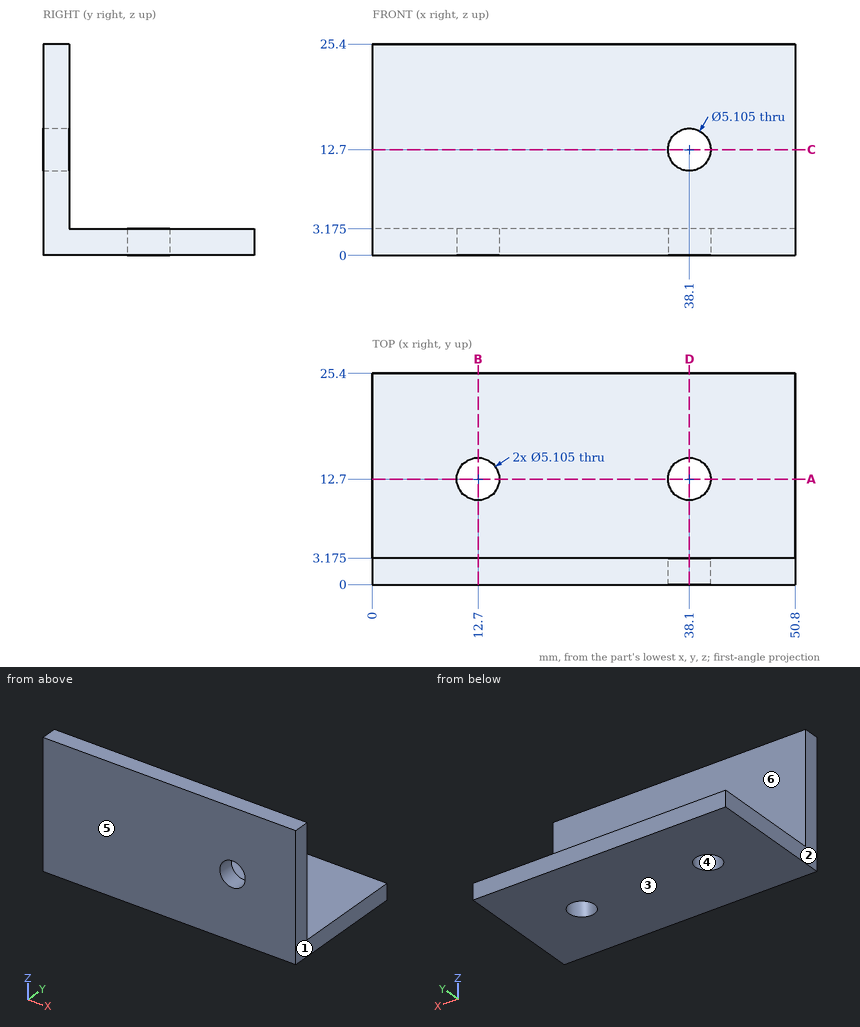
Input: dimensioned drawing with shaded views. Units: mm. Origin: part minimum x, y, z. A direction names the side the tool comes from. Give positions to 0.01 mm unless a question says otherwise; leave off trailing zeros. Loops run counter-clockwise (first coordinate to the right, second up) from the corner with the lowest first, then second, coordinate; pieces in that order, holes last. Notation, with made-up numbers: M 37.5,13.25 L 71.5,13.25 A19 cw 71.5,40.25 Z; hole C 25,68.25 d6. An arc over 180 degrees is marked long. Put each result on its own line as item: value. Start each with the question number.
1) Pull-direction query (X, two-part tool) for the marked faces 1, 2, 3 and 4; classes: pulls with the +X half, pulls with the -X half, needs draft (parallel to the pull), parting line crosses it, or undercut.
2) Cut plane A-A (y = 12.7). Output: boundary loops of the cut face in (x, z) (1 decimal), then the cut area to 3 significant figures.
3) Cut plane C-C (z = 12.7). Output: boundary loops of the cut face in (x, y) (1 decimal).
4) Cut plane D-D (x = 38.1). Output: boundary loops of the cut face in (y, z) (1 decimal), then the cut area to 3 significant figures.
5) Contact query for flat-ended pins moving along their axis: pin 1 (2 mm diameter, centred on x = 38, y = 6, fed in from +Z) (3 decimals); pin 2 (8 mm diameter, centred on y = 5.5, z = 18, fed in from -X); pin 3 (1 mm diameter, centred on y = 16, z = 4.5, fed in from +X); pin 4 (1 mm diameter, centred on x = 43, z = 14, fed in from +Y) (3 decimals). Output: stop coordinate, or through.
6) Cut plane B-B (x = 12.7). Output: boundary loops of the cut face in (y, z) (1 decimal).
7) Ray query, line 1 along Y through (x, z) = (38.1, 2); line 2 along Z through (x, y) = (41, 23.75) (1 decimal). Return the intervals inside material, ascending.
8) Access query for the marked faces 5 and 6. Directions: +Z, -Z, +X, -X, +Y, -Y. A direction counts if a zero-diameter tool reaches every point of the face in a straight line with its end or side. Return the directions, or none.
Verdict:
1. face 1: pulls with the +X half
1. face 2: pulls with the -X half
1. face 3: needs draft
1. face 4: undercut
2. outline: M 0,0 L 10.1,0 L 10.1,3.2 L 0,3.2 Z; M 15.3,0 L 35.5,0 L 35.5,3.2 L 15.3,3.2 Z; M 40.7,0 L 50.8,0 L 50.8,3.2 L 40.7,3.2 Z
2. area: 129 mm2
3. outline: M 0,0 L 35.5,0 L 35.5,3.2 L 0,3.2 Z; M 40.7,0 L 50.8,0 L 50.8,3.2 L 40.7,3.2 Z
4. outline: M 0,0 L 10.1,0 L 10.1,3.2 L 3.2,3.2 L 3.2,10.1 L 0,10.1 Z; M 0,15.3 L 3.2,15.3 L 3.2,25.4 L 0,25.4 Z; M 15.3,0 L 25.4,0 L 25.4,3.2 L 15.3,3.2 Z
4. area: 119 mm2
5. pin 1: z = 3.175
5. pin 2: x = 0
5. pin 3: through
5. pin 4: y = 3.175
6. outline: M 0,0 L 10.1,0 L 10.1,3.2 L 3.2,3.2 L 3.2,25.4 L 0,25.4 Z; M 15.3,0 L 25.4,0 L 25.4,3.2 L 15.3,3.2 Z
7. line 1: 0 to 10.15, 15.25 to 25.4
7. line 2: 0 to 3.2
8. face 5: +Z, -Z, +X, -X, -Y
8. face 6: +Z, +X, -X, +Y
